Here's how the part is built. I have some questions about the finished solid (model axes, mm). A direction names the side the tool comes from. Give positions to 0.01 mm unless a question says otherwise; leave off trailing zeros. Write each loop counter-clockwise with the first axis right and the second up, starting at its lowest first coordinate (ties: lowest second). Pieces come first, ordered by that corner, then holes. Notation, with made-up numbers: (-16.5, 60.5) -> (18.5, 60.5) arc R20 cw to (18.5, 81.5) -> close; hole circle Ø2 at (29, -11). An arc over 180 degrees is marked (long way). Use CSV: the item, a comma, the result in double quotes. Start each with the question number.
(1) For pin 1 Ø1 at (x, z) = (-5, 1) entering from +Y; pin 2 Ø2 at (x, y) = (-4, 1) entering from -Z, each with a flat end and sliding along its axis, tell me the tip position at first contact or that it passes through.
(2) Suppose I cut it at A-A on z = 0. List the corners of the cut face in (x, y) for me, plus the area to 3 significant figures.
(3) I need wall thicknesses on L1, parallel to Z at x = -3.25, y = 0.1; L2, parallel to Y at x = -4, z = -0.75; L3, parallel to X at y = 0.9, z = -1.05. Which ranges of each line are inside material? Lowest first, please. Write a range as [from, to].
(4) Which directions (+Z, -Z, +X, -X, +Y, -Y) give clear straight access to the entire face, cutting with the end or side of a thin tool? Please do faces 1 (the cylindrical face through (3.66, -0.27, -1.22)), 2 (the flat face through (-1.5, -1, 0)), 3 (the flat face through (-4, -0.75, 0)).
(5) Suppose I cut it at B-B on y = 0. List the corners of the cut face in (x, z) for me.
(6) Suppose I cut it at D-D on z = 1.45. List the corners of the cut face in (x, y) for me.
(7) Suppose I cut it at C-C on x = -1. List the corners of the cut face in (y, z) for me, plus the area to 3 significant figures.
Autodesk Inventor part; units mm, degrees
ref_plane "YZ Plane" through (0, 0, 0) normal (1, 0, 0) x (0, 1, 0)
ref_plane "XZ Plane" through (0, 0, 0) normal (0, 1, 0) x (-1, 0, 0)
ref_plane "XY Plane" through (0, 0, 0) normal (0, 0, 1) x (1, 0, 0)
sketch "Sketch1" plane through (0, 0, 0) normal (0, 0, 1) x (1, 0, 0)
  line L0 (-7.5, 0) -> (7.5, 0)
  line L1 (-7.5, 0) -> (-7.5, 1)
  line L2 (-7.5, 1) -> (-6, 1)
  line L3 (-6, 1) -> (-6, 1.25)
  line L4 (-6, 1.25) -> (-5.75, 1.25)
  line L5 (-5.75, 1.25) -> (-5.75, 1.75)
  line L6 (1.25, 1.25) -> (6, 1.25)
  line L7 (6, 1.25) -> (6, 1)
  line L8 (6, 1) -> (7.5, 1)
  line L9 (7.5, 1) -> (7.5, 0)
  line L10 (0, 0) -> (0, -6.3915) construction
  line L11 (-5.75, 1.75) -> (-1.5, 1.75)
  line L12 (-1.5, 1.75) -> (-1.5, 2)
  line L13 (-1.5, 2) -> (1.25, 2)
  line L14 (1.25, 2) -> (1.25, 1.25)
  dimension "d0" = 15
  dimension "d1" = 1.5
  dimension "d2" = 2
  dimension "d3" = 2.5
  dimension "d8" = 0.25
  dimension "d9" = 3.5
  dimension "d10" = 4
  dimension "d11" = 4.25
  dimension "d12" = 6.25
revolve "Revolution1" add sketch "Sketch1" angle 360 about axis through (-7.5, 0, 0) along (1, 0, 0)
sketch "Sketch2" plane through (-7.5, 0, 0) normal (-1, 0, 0) x (0, 0, 1)
  circle A0 centre (0, 0) radius 2
  line L0 (-1.854, -0.75) -> (1.854, -0.75)
  point P0 (0, 0)
  dimension "d13" = 0.75
extrude "Extrusion1" cut sketch "Sketch2" against normal up to surface (6 mm away) contours L0 A0 picked at (0, -1.1667)
properties part number "IP axle" material "Stainless Steel"
Geometry says:
1,pin 1,"y = 1.68"
1,pin 2,"z = -1.75"
2,outline,"(-7.5, -0.75) -> (-1.5, -0.75) -> (-1.5, -2) -> (1.25, -2) -> (1.25, -1.25) -> (6, -1.25) -> (6, -1) -> (7.5, -1) -> (7.5, 1) -> (6, 1) -> (6, 1.25) -> (1.25, 1.25) -> (1.25, 2) -> (-1.5, 2) -> (-1.5, 1.75) -> (-5.75, 1.75) -> (-5.75, 1.25) -> (-6, 1.25) -> (-6, 1) -> (-7.5, 1) -> close"
2,area,"39.6 mm²"
3,L1,"[-1.75, 1.75]"
3,L2,"[-0.75, 1.58]"
3,L3,"[-5.75, 1.25]"
4,face 1,"+X"
4,face 2,"-X"
4,face 3,"+Z, -Z, -X, -Y"
5,outline,"(-7.5, -1) -> (-6, -1) -> (-6, -1.25) -> (-5.75, -1.25) -> (-5.75, -1.75) -> (-1.5, -1.75) -> (-1.5, -2) -> (1.25, -2) -> (1.25, -1.25) -> (6, -1.25) -> (6, -1) -> (7.5, -1) -> (7.5, 1) -> (6, 1) -> (6, 1.25) -> (1.25, 1.25) -> (1.25, 2) -> (-1.5, 2) -> (-1.5, 1.75) -> (-5.75, 1.75) -> (-5.75, 1.25) -> (-6, 1.25) -> (-6, 1) -> (-7.5, 1) -> close"
6,outline,"(-5.75, -0.75) -> (-1.5, -0.75) -> (-1.5, -1.38) -> (1.25, -1.38) -> (1.25, 1.38) -> (-1.5, 1.38) -> (-1.5, 0.98) -> (-5.75, 0.98) -> close"
7,outline,"circle Ø4 at (0, 0)"
7,area,"12.6 mm²"
